```python
from build123d import *

# Parameters (mm, degrees)
F1_DEPTH = 101.6
F2_DEPTH = 50.8
F3_T     = -10.16
F4_R     = 5.07999


# Not quite as in the source:
# - a fillet or chamfer is up to 0.001 mm smaller than in the source, because OpenCascade refuses the exact size


with BuildPart() as f1:
    # F0 (on Front) → F1 (new body)
    with BuildSketch(Plane.XZ):
        Polygon((0, 43.6448735309), (0, 0), (50.223051581, 0), (50.8, 0), (50.8, 76.2), (0, 76.2), align=None)
    extrude(amount=F1_DEPTH)

    # F0 (on Front) → F2 (join)
    with BuildSketch(Plane.XZ):
        Polygon((50.223051581, 0), (0, 0), (0, 43.6448735309), (-24.9360222917, 43.7942571525), (-50.3949503798, 0.3018998023), (-25.4589280881, -43.4923573502), (24.9360222917, -43.7942571525), (50.3949503798, -0.3018998023), align=None)
    extrude(amount=F2_DEPTH)

    # F3: a shell. OpenCascade refuses it in one call, so the cavity is built on its own and cut out:
    # the body offset inwards by the wall thickness, plus a prism from it out through each open face.
    f3_core = offset(f1.part, amount=F3_T, kind=Kind.INTERSECTION, mode=Mode.PRIVATE)
    f3_exits = [f3_core.faces().sort_by_distance(p)[0] for p in [
        (25.4, -91.44, 38.1),
        (-1.965126, -40.64, -2.131269),
    ]]
    add(f3_core, mode=Mode.SUBTRACT)
    extrude(f3_exits, amount=-F3_T, mode=Mode.SUBTRACT)

    # F4 (radius 5.08 in the source; OpenCascade refuses exactly that, so slightly less here)
    f4_edges = [f1.edges().sort_by_distance(p)[0] for p in [
        (25.4, -101.6, 66.04),
        (40.64, -101.6, 38.1),
        (25.4, -101.6, 10.16),
        (10.16, -101.6, 38.1),
        (-28.897258, -50.8, 16.91546),
        (-29.097847, -50.8, -16.56803),
        (-0.200589, -50.8, -33.48349),
        (28.897258, -50.8, -16.91546),
        (-12.468011, -50.8, 43.719565),
        (-37.665486, -50.8, 22.048078),
        (-37.926939, -50.8, -21.595229),
        (-0.261453, -50.8, -43.643307),
        (37.665486, -50.8, -22.048078),
        (0, -101.6, 38.1),
        (25.4, -101.6, 76.2),
        (50.8, -101.6, 38.1),
        (25.4, -101.6, 0),
        (-9.565556, -50.8, 33.541995),
    ]]
    fillet(f4_edges, radius=F4_R)


solid = f1.part
```
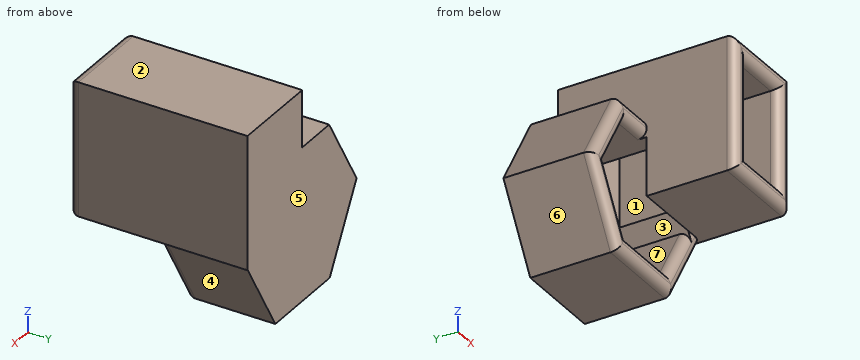
Geometry: final body of the model. Coordinates: model frame, mm. Face numbers are marked on the shaded views. A direction names the side the tool comes from. Round coordinates to 2 decimals unless told otherwise and drop trailing zeros. Loops run counter-clockwise (first coordinate to the right, second up) from the corner with the lowest first, then second, coordinate; pieces in that order, holes last. Notation, with made-up numbers: (-3.75, -12) -> (26.25, -12) arc R27 ccw to (26.25, 26) -> close; hole circle Ø7 at (-19.75, 30). An arc over 180 degrees is marked (long way). Use one line per item in the form item = value. Start each with the question number.
1) Line query: L1, parallel to Z at x = 37.5, y = -83; L2, parallel to X at y = -59, z = 36; L3, parallel to X at y = -97, z = 54.5. Output: solid intervals per line, ascending.
2) Section A-A on y = -65. Output: boundary loops of the cut face in (x, z), then the cut area to 3 significant figures.
3) Section D-D on y = -19.5. Output: boundary loops of the cut face in (x, z).
4) Section C-C on y = -6.5. Output: boundary loops of the cut face in (x, z), then the cut area to 3 significant figures.
5) Draft query along X for the marked faces 4, 5, 6 and 7. Return one class per face: released by +X, released by -X, zero draft, split by the parting line, or undercut.
6) Access query for the marked faces 1, 2 and 3. Directions: +Z, -Z, +X, -X, +Y, -Y. A direction counts if a zero-diameter tool reaches every point of the face in a straight line with its end or side. Return the directions, or none.
7) First-contact query: P1, Ø15, axis at x = 33.5, y = -71.5, coming from the -Z side; P2, Ø1, axis at x = 14.5, z = 43.5, coming from the -Y side; P3, Ø1.5, axis at x = -25, y = -14.5, coming from the +Z side. Flat tips, straight axial feed; report the tip coordinate or a pass-through.
Response:
q1.L1 = 0 to 10.16, 66.04 to 76.2
q1.L2 = 0 to 10.16, 40.64 to 50.8
q1.L3 = 0.02 to 10.14, 40.66 to 50.78
q2.outline = (0, 0) -> (50.8, 0) -> (50.8, 76.2) -> (0, 76.2) -> close; hole (10.16, 10.16) -> (40.64, 10.16) -> (40.64, 66.04) -> (10.16, 66.04) -> close
q2.area = 2,170 mm^2
q3.outline = (-50.39, 0.3) -> (-25.46, -43.49) -> (24.94, -43.79) -> (50.39, -0.3) -> (50.22, 0) -> (50.8, 0) -> (50.8, 76.2) -> (0, 76.2) -> (0, 43.64) -> (-24.94, 43.79) -> close; hole (-38.66, 0.23) -> (-19.53, -33.37) -> (19.13, -33.6) -> (38.66, -0.23) -> (32.75, 10.16) -> (40.64, 10.16) -> (40.64, 66.04) -> (10.16, 66.04) -> (10.16, 33.42) -> (-19.13, 33.6) -> close
q4.outline = (-50.39, 0.3) -> (-25.46, -43.49) -> (24.94, -43.79) -> (50.39, -0.3) -> (50.22, 0) -> (50.8, 0) -> (50.8, 76.2) -> (0, 76.2) -> (0, 43.64) -> (-24.94, 43.79) -> close
q4.area = 8,820 mm^2
q5.face_4 = released by +X
q5.face_5 = zero draft
q5.face_6 = released by -X
q5.face_7 = undercut
q6.face_1 = -Y
q6.face_2 = +Z, +X, -X, +Y, -Y
q6.face_3 = none
q7.P1 = 0
q7.P2 = -10.16
q7.P3 = 43.79
